Design review of the part shown in the three views and the two pictorial views. Dimensions are in mm from the part's minimum x, y and z. A direction names the side the tool comes from. Round coordinates to 2 decimals unless told otherwise and drop trailing zeros. Write each loop counter-clockwise with the first axis right and the second up, starting at its lowest first coordinate (ties: lowest second). Pieces come first, ordered by that corner, then holes. Notation, with made-up numbers: (59, 85) -> (65, 85) arc R12 ccw to (65, 93) -> close; hole circle Ø3 at (13.25, 12). An arc over 180 degrees is marked (long way). Answer as a JSON object with one key per item and string values. Group by question number.
1) Machinability: for the marked faces 1, 2 and 3, which of the approach directions +Z, -Z, +X, -X, +Y, -Y give a long, thin tool a straight path to every point of the face, cutting with its end or side? Answer none if there is none.
2) Insertion check: pin 1 Ø3 at (y, z) = (3.5, 17) entering from -X; pin 2 Ø6 at (y, z) = (7, 158.5) entering from +X; pin 3 Ø1 at (x, y) = (58.5, 10) entering from -Z. Each pin has a flat end and moves straight along its axis. Give the tip position at first contact, or say it passes through.
3) We need section B-B, the plane x = 98. Write out the cut boundary in (y, z).
4) We need section A-A, the plane y = 10. Write out the cut boundary in (x, z), then the cut area to 3 significant figures.
5) We need section C-C, the plane z = 123. Write out the cut boundary in (x, y), then the cut area to 3 significant figures.
6) To check wall thickness, follow probe 1 along X at (y, z) = (4.5, 116); probe 2 along Z at (x, y) = (72, 1.75); probe 3 along X at (y, z) = (10.75, 53). State the ranges of each line that lie inside material, in increasing order. Write a range as [from, to].
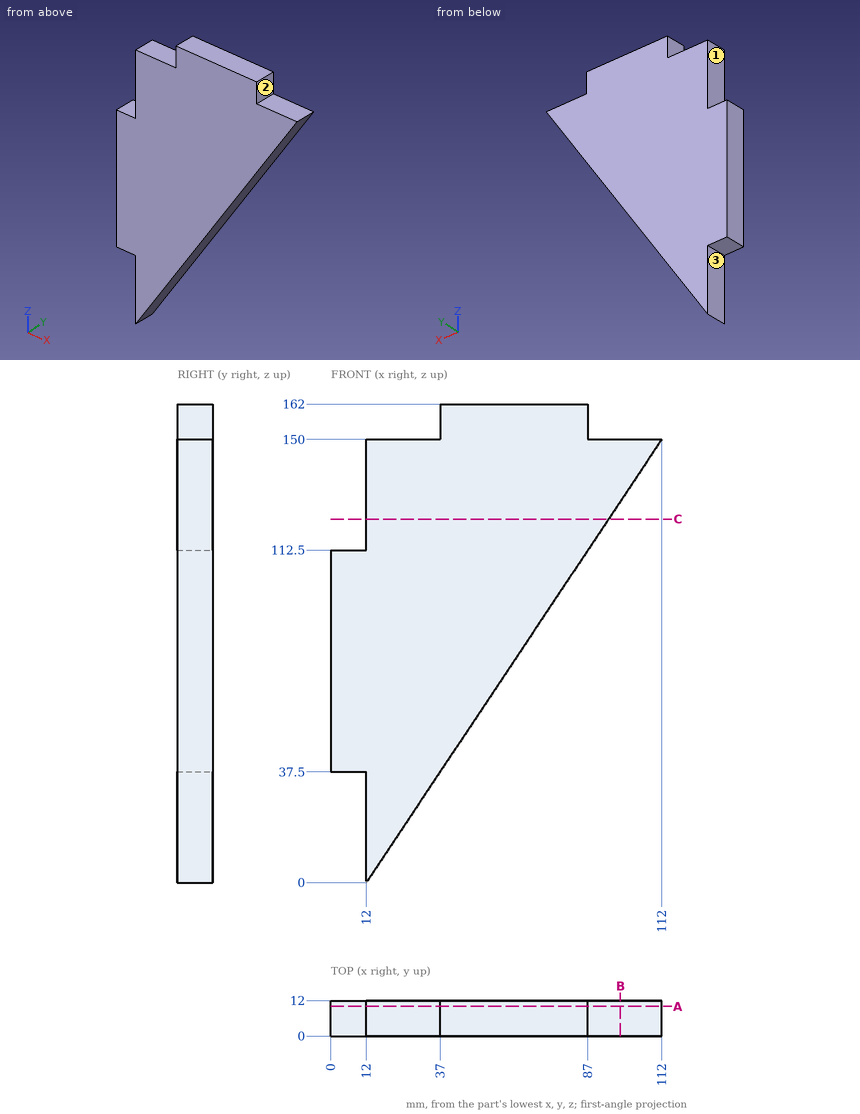
Here are the results:
{
 "1": {"face 1": "+Z, -X, +Y, -Y", "face 2": "+Z, +X, +Y, -Y", "face 3": "-Z, -X, +Y, -Y"},
 "2": {"pin 1": "stops at x = 12", "pin 2": "stops at x = 87", "pin 3": "stops at z = 69"},
 "3": {"outline": "(0, 129) -> (12, 129) -> (12, 150) -> (0, 150) -> close"},
 "4": {"outline": "(0, 37.5) -> (12, 37.5) -> (12, 0) -> (112, 150) -> (87, 150) -> (87, 162) -> (37, 162) -> (37, 150) -> (12, 150) -> (12, 112.5) -> (0, 112.5) -> close", "area": "9,000 mm^2"},
 "5": {"outline": "(12, 0) -> (94, 0) -> (94, 12) -> (12, 12) -> close", "area": "984 mm^2"},
 "6": {"probe 1": "x = [12, 89.33]", "probe 2": "z = [90, 162]", "probe 3": "x = [0, 47.33]"}
}
